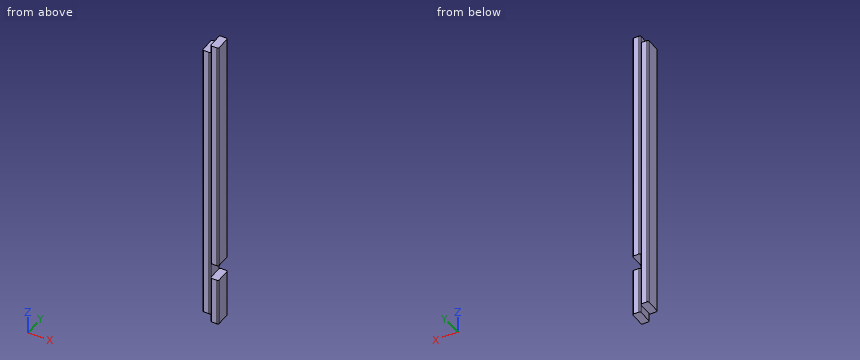
```python
from build123d import *

# Parameters (mm, degrees)
F1_DEPTH = 723.9
F2_DEPTH = 704.85
F3_DEPTH = 19.05
F4_W     = 3.1496
F4_H     = 38.1
F4_W_2   = 12.7508
F5_DEPTH = 38.101


# Not quite as in the source:
# - a feature names something its author has since deleted; it is built from what else it names


with BuildPart() as f1:
    # F0 (on Top) → F1 (new body)
    with BuildSketch(Plane.XY):
        with BuildLine():
            Line((19.05, 34.9504), (19.05, 3.1496))
            ThreePointArc((19.05, 3.1496), (19.972496482, 0.922496482), (22.1996, 0))
            Line((22.1996, 0), (34.9504, 0))
            ThreePointArc((34.9504, 0), (37.177503518, 0.922496482), (38.1, 3.1496))
            Line((38.1, 3.1496), (38.1, 34.9504))
            ThreePointArc((38.1, 34.9504), (37.177503518, 37.177503518), (34.9504, 38.1))
            Line((34.9504, 38.1), (22.1996, 38.1))
            ThreePointArc((22.1996, 38.1), (19.972496482, 37.177503518), (19.05, 34.9504))
        make_face()
    extrude(amount=F1_DEPTH)

    # F0 (on Top) → F2 (join)
    with BuildSketch(Plane.XY):
        with BuildLine():
            ThreePointArc((0, 3.1496), (0.922496482, 0.922496482), (3.1496, 0))
            Line((3.1496, 0), (15.9004, 0))
            ThreePointArc((15.9004, 0), (18.127503518, 0.922496482), (19.05, 3.1496))
            Line((19.05, 3.1496), (19.05, 34.9504))
            ThreePointArc((19.05, 34.9504), (18.127503518, 37.177503518), (15.9004, 38.1))
            Line((15.9004, 38.1), (3.1496, 38.1))
            ThreePointArc((3.1496, 38.1), (0.922496482, 37.177503518), (0, 34.9504))
            Line((0, 34.9504), (0, 3.1496))
        make_face()
        with BuildLine():
            Line((19.05, 34.9504), (19.05, 3.1496))
            ThreePointArc((19.05, 3.1496), (19.972496482, 0.922496482), (22.1996, 0))
            Line((22.1996, 0), (34.9504, 0))
            ThreePointArc((34.9504, 0), (37.177503518, 0.922496482), (38.1, 3.1496))
            Line((38.1, 3.1496), (38.1, 34.9504))
            ThreePointArc((38.1, 34.9504), (37.177503518, 37.177503518), (34.9504, 38.1))
            Line((34.9504, 38.1), (22.1996, 38.1))
            ThreePointArc((22.1996, 38.1), (19.972496482, 37.177503518), (19.05, 34.9504))
        make_face()
    extrude(amount=F2_DEPTH)

    # F0 (on Top) → F3 (cut)
    with BuildSketch(Plane.XY):
        with BuildLine():
            ThreePointArc((0, 3.1496), (0.922496482, 0.922496482), (3.1496, 0))
            Line((3.1496, 0), (15.9004, 0))
            ThreePointArc((15.9004, 0), (18.127503518, 0.922496482), (19.05, 3.1496))
            Line((19.05, 3.1496), (19.05, 34.9504))
            ThreePointArc((19.05, 34.9504), (18.127503518, 37.177503518), (15.9004, 38.1))
            Line((15.9004, 38.1), (3.1496, 38.1))
            ThreePointArc((3.1496, 38.1), (0.922496482, 37.177503518), (0, 34.9504))
            Line((0, 34.9504), (0, 3.1496))
        make_face()
    extrude(amount=F3_DEPTH, mode=Mode.SUBTRACT)

    # F4 (on face) → F5 (cut, through all)
    with BuildSketch(Plane.XZ):
        with Locations((36.5252, 133.35)):
            Rectangle(F4_W, F4_H)
        with Locations((28.575, 133.35)):
            Rectangle(F4_W_2, F4_H)
        with Locations((20.6248, 133.35)):
            Rectangle(F4_W, F4_H)
    extrude(amount=-F5_DEPTH, mode=Mode.SUBTRACT)


solid = f1.part
```
Input: part model. Units: mm. Frame: model coordinates. Coordinates: 2 decimals unless noted, no trailing zeros. Write each loop counter-clockwise with the first axis right and the second up, starting at its lowest first coordinate (ties: lowest second). Pieces come first, ordered by that corner, then holes.
1) Pin query (flat end, axial travel): pin 1 Ø9.5 at (y, z) = (20.5, 10) entering from -X; pin 2 Ø5.5 at (x, y) = (5, 24.5) entering from +Z; pin 3 Ø9.5 at (x, y) = (5.5, 14.5) entering from -Z; pin 4 Ø12 at (x, z) = (17, 528) entering from -Y. Return the tip coordinate at first contact, or that it passes through.
2) Section A-A on y = 21.5. Output: boundary loops of the cut face in (x, z).
3) Material intervals for line 1 along Z through (x, y) = (24, 35); line 2 along X through (y, z) = (36, 605.5); line 3 along Z through (x, y) = (16, 19), sorted ascending.
4) Section B-B on x = 10. Output: boundary loops of the cut face in (y, z).
Check result:
1. pin 1: stops at x = 19.05
1. pin 2: stops at z = 704.85
1. pin 3: stops at z = 19.05
1. pin 4: stops at y = 0
2. outline: (0, 19.05) - (19.05, 19.05) - (19.05, 0) - (38.1, 0) - (38.1, 114.3) - (19.05, 114.3) - (19.05, 152.4) - (38.1, 152.4) - (38.1, 723.9) - (19.05, 723.9) - (19.05, 704.85) - (0, 704.85) - close
3. line 1: z = 0 to 114.3, 152.4 to 723.9
3. line 2: x = 0.18 to 18.87, 19.23 to 37.92
3. line 3: z = 19.05 to 704.85
4. outline: (0, 19.05) - (38.1, 19.05) - (38.1, 704.85) - (0, 704.85) - close
